The listing builds one solid part. Answer for the finished solid, in the listing's coordinates (mm). A direction names the side the tool comes from. Round coordinates to 2 decimals unless told otherwise and drop trailing zeros. Write each loop counter-clockwise with the first axis right and the second up, starting at its lowest first coordinate (ties: lowest second). Pieces come first, ordered by that corner, then holes.
Item 1: A tool of negligible diameter and unlimited length cuts with its end or side. For faces 4 (the face through (0, 0, -6)), 5 (the face through (-44, -1, -6)), 6 (the face through (-20, 0, -8.5)), 7 (the face through (34.078, -3.615, -5.67)), from which of +Z, -Z, +X, -X, +Y, -Y can it reach the whole face along a straight path? Write none if from no direction.
Item 2: Find section A-A on z = -1. Give the vertices of the cut face in (x, y) (3 decimals).
Item 3: Find section B-B on y = 0. Give the number of separate pieces and of enclosed holes in the cut face, then the cut area to 3 significant figures.
Item 4: Find the intervals of material crossed by probe 1 along X at (y, z) = (0.5, -4); probe 2 along Y at (x, z) = (20.75, -6); probe 3 along X at (y, z) = (-2.5, -4.75), in increasing order.
Item 5: For a pull along Z with two mould halves and no side action, classify faces 1 (the face through (14, 0.9, -7.2)), 2 (the face through (-41.467, 0.421, -2.958)), 3 (the face through (-4, 0, 0)) as +Z half, -Z half, draft (parallel to the pull), parting line (faces both ways), or undercut.
Item 6: Find section C-C on y = -7. Give the vertices of the cut face in (x, z).
Item 7: Find section D-D on x = -14.5. Give the vertices of the cut face in (y, z), then the cut area to 3 significant figures.
Item 8: Each of these flat-tipped pins is pushed along its axis until it touches: pin 1 (1 mm diameter, centred on x = 1.5, z = -9.5, fed in from +Y); pin 2 (3.5 mm diameter, centred on y = 0, z = -6, fed in from +X); pin 3 (2 mm diameter, centred on y = 3.5, z = -1.5, fed in from -X); pin 4 (2 mm diameter, centred on x = -42.8, y = 0, fed in from +Z). Where does it stop, or does it pass through?
```python
from build123d import *

# Parameters (mm, degrees)
SKETCH_1_R               = 1.400000008
SKETCH_1_R_2             = 4.074999999
EXTRUDE_1_DEPTH          = 11.500000001
SKETCH_2_R               = 1.499999995
CUT_EXTRUDE_1_DEPTH      = 52.126386943
CUT_EXTRUDE_START        = 40
SKETCH_2_3_R             = 3.099999995
CUT_EXTRUDE_2_DEPTH      = 12.126386986
CUT_EXTRUDE_3_DEPTH      = 52.126386986
CUT_EXTRUDE_3_DEPTH_BACK = 52.126386986
SKETCH_4_R               = 2.999999992
CUT_EXTRUDE_4_DEPTH      = 2.5


with BuildPart() as part:
    # Эскиз1 → Бобышка-Вытянуть1 (new body)
    with BuildSketch(Plane.XY):
        with BuildLine():
            Line((-43.122227837, -5.991460588), (31.66443883, -9.985767648))
            ThreePointArc((31.66443883, -9.985767648), (42.197772163, 2e-09), (31.66443883, 9.985767652))
            Line((31.66443883, 9.985767652), (-43.122227837, 5.991460592))
            ThreePointArc((-43.122227837, 5.991460592), (-48.802227837, 2e-09), (-43.122227837, -5.991460588))
        make_face()
        with Locations((-42.802227837, 2e-09)):
            Circle(SKETCH_1_R, mode=Mode.SUBTRACT)
        with Locations((32.197772163, 2e-09)):
            Circle(SKETCH_1_R_2, mode=Mode.SUBTRACT)
    extrude(amount=-EXTRUDE_1_DEPTH)

    # Эскиз2 → Вырез-Вытянуть1 (cut, through all)
    with BuildSketch(Plane(origin=(0, 0, 0), x_dir=(0, 0, -1), z_dir=(1, 0, 0))):
        with Locations(Location((6, 6e-09, 0), (0, 0, 180))):
            Circle(SKETCH_2_R)
    extrude(amount=CUT_EXTRUDE_1_DEPTH, mode=Mode.SUBTRACT)

    # Эскиз2<3> → Вырез-Вытянуть2 (cut, through all)
    with BuildSketch(Plane(origin=(0, 0, 0), x_dir=(0, 0, -1), z_dir=(1, 0, 0)).offset(CUT_EXTRUDE_START)):
        with Locations(Location((6, 6e-09, 0), (0, 0, 180))):
            Circle(SKETCH_2_3_R)
    extrude(amount=CUT_EXTRUDE_2_DEPTH, mode=Mode.SUBTRACT)

    # Эскиз3 → Вырез-Вытянуть3 (cut, two sides: drawn at the far end of the back side and taken through both)
    with BuildSketch(Plane(origin=(0, 0, 0), x_dir=(1, 0, 0), z_dir=(0, 1, 0)).offset(-CUT_EXTRUDE_3_DEPTH_BACK)):
        with BuildLine():
            Line((-57.148549842, 26.385379488), (0, 26.385379488))
            Line((0, 26.385379488), (0, 11.5))
            ThreePointArc((0, 11.5), (-0.878679656, 9.378679656), (-3, 8.5))
            Line((-3, 8.5), (-57.148549842, 8.5))
            Line((-57.148549842, 8.5), (-57.148549842, 26.385379488))
        make_face()
    extrude(amount=CUT_EXTRUDE_3_DEPTH + CUT_EXTRUDE_3_DEPTH_BACK, mode=Mode.SUBTRACT)

    # Эскиз4 → Вырез-Вытянуть4 (cut)
    with BuildSketch(Plane(origin=(0, 0, -8.5), x_dir=(-1, 0, 0), z_dir=(0, 0, -1))):
        with Locations((42.802227837, 2e-09)):
            Circle(SKETCH_4_R)
    extrude(amount=-CUT_EXTRUDE_4_DEPTH, mode=Mode.SUBTRACT)


solid = part.part
```
Check values:
1. face 4: +X
1. face 5: -Z
1. face 6: -Z, -X, +Y, -Y
1. face 7: +Z, -Z
2. outline: (-43.122, -5.991) - (31.664, -9.986) arc R10 ccw (long way) to (31.664, 9.986) - (-43.122, 5.991) arc R6 ccw to start; hole circle Ø2.8 at (-42.802, 0); hole circle Ø8.15 at (32.198, 0)
3. separate pieces: 4
3. enclosed holes: 0
3. area: 667 mm2
4. probe 1: x = -48.78 to -44.11, -41.49 to 28.15, 36.24 to 40
4. probe 2: y = -9.4 to -1.5, 1.5 to 9.4
4. probe 3: x = -48.26 to 28.98, 35.42 to 40
5. face 1: undercut
5. face 2: draft
5. face 3: +Z half
6. outline: (-24.24, -8.5) - (-3, -8.5) arc R3 cw to (0, -11.5) - (39.34, -11.5) - (39.34, 0) - (-24.24, 0) - close
7. outline: (-7.52, -8.5) - (7.52, -8.5) - (7.52, 0) - (-7.52, 0) - close
7. area: 128 mm2
8. pin 1: stops at y = 8.4
8. pin 2: stops at x = 40
8. pin 3: stops at x = -48.26
8. pin 4: passes through
